from build123d import *

# Parameters (mm, degrees)
SKETCH4_W           = 140
SKETCH4_H           = 18
BOSS_EXTRUDE1_DEPTH = 86
BOSS_EXTRUDE3_DEPTH = 12
SKETCH6_5_R         = 25
SKETCH6_5_R_2       = 15
BOSS_EXTRUDE4_DEPTH = 35
SKETCH6_6_R         = 20
SKETCH6_6_R_2       = 10
BOSS_EXTRUDE5_DEPTH = 30
SKETCH11_R          = 5
CUT_EXTRUDE1_DEPTH  = 168.095780916
SKETCH12_W          = 60
SKETCH12_H          = 16.179667724
CUT_EXTRUDE2_DEPTH  = 207.448540804


with BuildPart() as part:
    # Sketch4 → Boss-Extrude1 (new body)
    with BuildSketch(Plane.XY):
        with Locations((0, -9)):
            Rectangle(SKETCH4_W, SKETCH4_H)
    extrude(amount=BOSS_EXTRUDE1_DEPTH)

    # Sketch6 → Boss-Extrude3 (add)
    with BuildSketch(Plane.XY):
        with BuildLine():
            Line((-70, 38), (-70, 0))
            Line((-70, 0), (70, 0))
            Line((70, 0), (44.294494718, 105.897247359))
            ThreePointArc((44.294494718, 105.897247359), (44.822997079, 102.969649142), (45, 100))
            ThreePointArc((45, 100), (20, 75), (-5, 100))
            Line((-5, 100), (-5, 83))
            ThreePointArc((-5, 83), (-12.32233047, 65.32233047), (-30, 58))
            Line((-30, 58), (-50, 58))
            ThreePointArc((-50, 58), (-35.857864376, 52.142135624), (-30, 38))
            ThreePointArc((-30, 38), (-50, 18), (-70, 38))
        make_face()
    extrude(amount=BOSS_EXTRUDE3_DEPTH)

    # Sketch6_5 → Boss-Extrude4 (add)
    with BuildSketch(Plane.XY):
        with Locations(Location((20, 100, 0), (0, 0, 180))):
            Circle(SKETCH6_5_R)
        with Locations((20, 100)):
            Circle(SKETCH6_5_R_2, mode=Mode.SUBTRACT)
    extrude(amount=BOSS_EXTRUDE4_DEPTH)

    # Sketch6_6 → Boss-Extrude5 (add)
    with BuildSketch(Plane.XY):
        with Locations(Location((-50, 38, 0), (0, 0, 180))):
            Circle(SKETCH6_6_R)
        with Locations((-50, 38)):
            Circle(SKETCH6_6_R_2, mode=Mode.SUBTRACT)
    extrude(amount=BOSS_EXTRUDE5_DEPTH)

    # Sketch11 → Cut-Extrude1 (cut, through all)
    with BuildSketch(Plane(origin=(0, 0, 0), x_dir=(1, 0, 0), z_dir=(0, 1, 0))):
        with Locations(Location((-55, -66, 0), (0, 0, 270))):
            Circle(SKETCH11_R)
        with Locations(Location((-55, -26, 0), (0, 0, 270))):
            Circle(SKETCH11_R)
        with Locations(Location((55, -26, 0), (0, 0, 270))):
            Circle(SKETCH11_R)
        with Locations(Location((55, -66, 0), (0, 0, 270))):
            Circle(SKETCH11_R)
    extrude(amount=-CUT_EXTRUDE1_DEPTH, mode=Mode.SUBTRACT)

    # Sketch12 → Cut-Extrude2 (cut, through all)
    with BuildSketch(Plane(origin=(70, 0, 0), x_dir=(0, 0, -1), z_dir=(1, 0, 0))):
        with Locations((-49.575704937, -24.089833862)):
            Rectangle(SKETCH12_W, SKETCH12_H)
    extrude(amount=-CUT_EXTRUDE2_DEPTH, mode=Mode.SUBTRACT)


solid = part.part
Check sheet for the modelled part. Datum: model origin and axes. Units: mm. A direction names the side the tool comes from. Give positions to 0.01 mm unless a question says otherwise; leave off trailing zeros. Loops run counter-clockwise (first coordinate to the right, second up) from the corner with the lowest first, then second, coordinate; pieces in that order, holes last. Notation, with made-up numbers: M -20.75,28.5 L -16.75,28.5 A30 ccw -16.75,60.5 Z; hole C 41.25,48.5 d2. An arc over 180 degrees is marked long. Use a Markdown table: item, result. Add a question column.
Q1. Sectioned sample at B-B, the plane z = 66. Record the cut outline in (x, y), then the cut area to 3 significant figures.
Q2. Sectioned sample at C-C, the plane x = -55. Record the cut outline in (y, z), then the cut area to 3 significant figures.
Q3. Mould release check, pull along Z, two halves, no side actions. Record for faces 1 (the flat face through (-41, 33, 30)), 2 (the cylindrical face through (-12.129, 65.518, 5.916)), 3 (the cylindrical face through (-50.043, -7.888, 25.349)): pulls with the +Z half, pulls with the -Z half, needs draft (parallel to the pull), parting line crosses it, or undercut.
Q4. Scan lines: line 1 along X through (y, z) = (-12.5, 26); line 2 along Y through (x, z) = (20, 25); line 3 along Y through (x, z) = (60, 16.5). Record each from-to range of solid material in increasing order. Write a range as [from, to].
Q5. Sectioned sample at D-D, the plane z = 5. Record the cut outline in (x, y).
Q6. Go/stop test with flat-tipped pins: pin 1 (23 mm diameter, centred on x = -50, y = 38, fed in from +Z); pin 2 (6 mm diameter, centred on x = -44, z = 6.5, fed in from +Y); pin 3 (1.6 mm diameter, centred on x = -17.5, y = -17.5, fed in from -Z); pin 4 (3 mm diameter, centred on x = -11.5, z = 59.5, fed in from +Y). Record where each tip stops, or that it passes through.
Q7. Sectioned sample at A-A, the plane x = 20. Record the cut outline in (y, z).
Q8. Tool access check on faces 4 (the cylindrical face through (25.42, 124.406, 21.144)), 5 (the flat face through (-1, 0, 48)), 6 (the flat face through (1, -16, 50)), 7 (the flat face through (9, 111, 35)). Record the directions out of +Z, -Z, +X, -X, +Y, -Y that give a thin tool (end or side, any length) a straight path to the whole face; none if there is none.
Verdict:
| question | item | result |
|---|---|---|
| 1 | outline | M -70,-16 L -60,-16 L -60,0 L -70,0 Z; M -50,-16 L 50,-16 L 50,0 L -50,0 Z; M 60,-16 L 70,-16 L 70,0 L 60,0 Z |
| 1 | area | 1,920 mm^2 |
| 2 | outline | M -18,0 L 29.34,0 L 29.34,30 L 18.64,30 L 18.64,12 L 0,12 L 0,21 L -16,21 L -16,19.58 L -18,19.58 Z; M -18,79.58 L -16,79.58 L -16,71 L 0,71 L 0,86 L -18,86 Z; M -16,31 L 0,31 L 0,61 L -16,61 Z; M 46.66,0 L 57.36,0 L 57.36,30 L 46.66,30 Z |
| 2 | area | 1,970 mm^2 |
| 3 | face 1 | pulls with the +Z half |
| 3 | face 2 | needs draft |
| 3 | face 3 | undercut |
| 4 | line 1 | [-70, -60], [-50, 50], [60, 70] |
| 4 | line 2 | [-16, 0], [75, 85], [115, 125] |
| 4 | line 3 | [-18, 0] |
| 5 | outline | M -70,-18 L 70,-18 L 70,0 L 44.29,105.9 A25 ccw -5,100 L -5,83 A25 cw -30,58 L -50,58 A20 ccw -70,38 Z; hole C -50,38 d20; hole C 20,100 d30 |
| 6 | pin 1 | z = 30 |
| 6 | pin 2 | y = 58 |
| 6 | pin 3 | z = 0 |
| 6 | pin 4 | y = 0 |
| 7 | outline | M -18,0 L 85,0 L 85,35 L 75,35 L 75,12 L 0,12 L 0,86 L -18,86 L -18,79.58 L -16,79.58 L -16,19.58 L -18,19.58 Z; M 115,0 L 125,0 L 125,35 L 115,35 Z |
| 8 | face 4 | +Z |
| 8 | face 5 | +Z, +X, -X |
| 8 | face 6 | +X, -X, -Y |
| 8 | face 7 | +Z, +X, -X, +Y |
